Here's how the part is built. I have some questions about the finished solid (model axes, mm). Face numbers are marked on the shaded views. Coordinates: 2 decimals unless noted, no trailing zeros. Write each loop counter-clockwise with the first axis right and the second up, starting at its lowest first coordinate (ties: lowest second). Pieces come first, ordered by that corner, then holes.
Item 1: I want a section at B-B (z = 74). Count the separate pieces of the cut face and the enclosed holes in it, and give its area (3 significant figures).
Item 2: I'm going to push flat-ended pins straight in: P1, Ø21, axis at x = 35.5, z = 55.5, coming from the +Y side; P2, Ø5, axis at y = -2, z = 46, coming from the +X side; P3, Ø5, axis at y = -7, z = 48.5, coming from the +X side. Where does each tip first touch, or does it pass through?
Item 3: I want a section at D-D (x = 32). Please give me the cut outline in (y, z).
Item 4: If we mould it in two halves opening along Y, with no side actions, what happens to the marked faces 1 and 2? For each: pulls with the +Y half, pulls with the -Y half, needs draft (parallel to the pull), parting line crosses it, or undercut.
Item 5: I want a section at A-A (x = 51.5). Please give me the cut outline in (y, z).
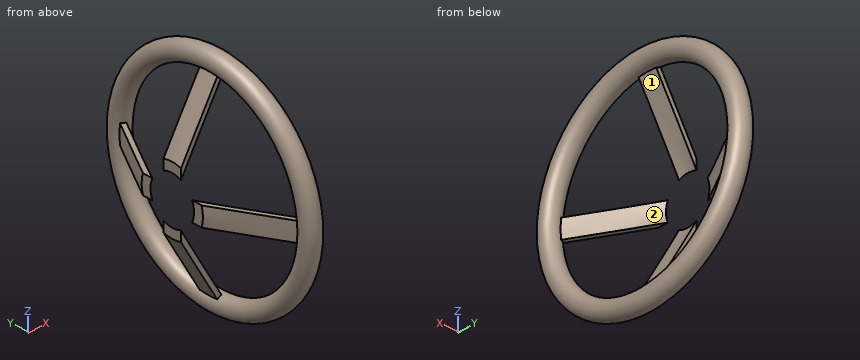
from build123d import *

# Parameters (mm, degrees)
F2_W     = 100
F2_H     = 100
F3_DEPTH = 100
F4_R     = 10
F6_W     = 96.7741915935
F6_H     = 197.4193443438
F7_DEPTH = 50


with BuildPart() as f1:
    # F0 (on Front) → F1 (revolve)
    with BuildSketch(Plane.XZ):
        Polygon((59.1784025919, 102.5), (0, 0), (5.7735026919, 0), (63.5085296109, 100), align=None)
    revolve(axis=Axis((20.5558100715, 0, 0), (1, 0, 0)))

    # F2 (on Right) → F3 (cut)
    with BuildSketch(Plane.YZ):
        with Locations((60, 60)):
            Rectangle(F2_W, F2_H)
        with Locations((60, -60)):
            Rectangle(F2_W, F2_H)
        with Locations((-60, 60)):
            Rectangle(F2_W, F2_H)
        with Locations((-60, -60)):
            Rectangle(F2_W, F2_H)
    extrude(amount=F3_DEPTH, mode=Mode.SUBTRACT)

    # F4 (on Front) → F5 (revolve)
    with BuildSketch(Plane.XZ):
        with Locations((65, 107.8704196738)):
            Circle(F4_R)
    revolve(axis=Axis((29.1963377967, 0, 0), (1, 0, 0)))

    # F6 (on Front) → F7 (cut, symmetric)
    with BuildSketch(Plane.XZ):
        with Locations((-28.3870957967, -5.0861872733)):
            Rectangle(F6_W, F6_H)
    extrude(amount=F7_DEPTH, both=True, mode=Mode.SUBTRACT)


solid = f1.part
Answer:
1. separate pieces: 3
1. enclosed holes: 0
1. area: 984 mm2
2. P1: stops at y = 10
2. P2: stops at x = 33.8
2. P3: stops at x = 35.51
3. outline: (-54.52, -10) - (-44.31, -10) arc R45.43 cw to (-44.31, 10) - (-54.52, 10) arc R55.43 ccw to start; (-10, -54.52) arc R55.43 ccw to (10, -54.52) - (10, -44.31) arc R45.43 cw to (-10, -44.31) - close; (-10, 44.31) arc R45.43 cw to (10, 44.31) - (10, 54.52) arc R55.43 ccw to (-10, 54.52) - close; (44.31, -10) - (54.52, -10) arc R55.43 ccw to (54.52, 10) - (44.31, 10) arc R45.43 cw to start
4. face 1: undercut
4. face 2: undercut
5. outline: (-88.64, -10) - (-78.57, -10) arc R79.2 cw to (-78.57, 10) - (-88.64, 10) arc R89.2 ccw to start; (-10, -88.64) arc R89.2 ccw to (10, -88.64) - (10, -78.57) arc R79.2 cw to (-10, -78.57) - close; (-10, 78.57) arc R79.2 cw to (10, 78.57) - (10, 88.64) arc R89.2 ccw to (-10, 88.64) - close; (78.57, -10) - (88.64, -10) arc R89.2 ccw to (88.64, 10) - (78.57, 10) arc R79.2 cw to start
